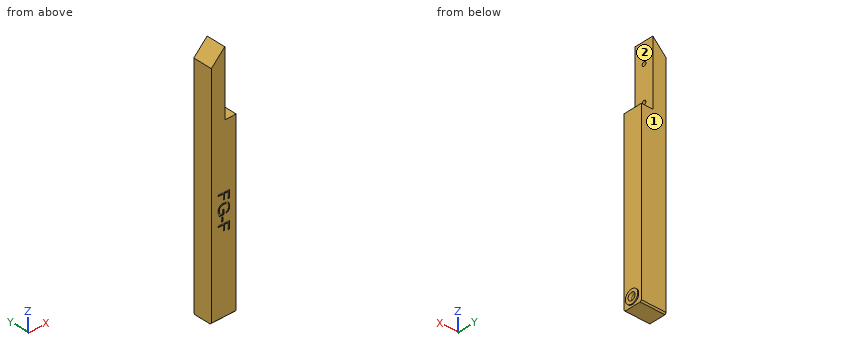
```python
from build123d import *

# Parameters (mm, degrees)
ESQUISSE1_W                         = 13
ESQUISSE1_H                         = 126
BOSS_EXTRU_1_DEPTH                  = 10
ESQUISSE2_W                         = 6
ESQUISSE2_H                         = 34
ENL_V_MAT_EXTRU_1_DEPTH             = 155.389928428
ENL_V_START                         = 1.2
ENL_V_MAT_EXTRU_2_DEPTH             = 0.4
ENL_V_MAT_EXTRU_3_DEPTH             = 0.4
ENL_V_MAT_EXTRU_4_DEPTH             = 0.4
ESQUISSE6_W                         = 0.740791559
ESQUISSE6_H                         = 2.263300419
ENL_V_MAT_EXTRU_5_DEPTH             = 0.4
D_POUILLE1_ANGLE                    = -0.092269995
D_POUILLE2_ANGLE                    = 0.092269995
D_POUILLE3_ANGLE                    = -45
ESQUISSE7_W                         = 0.5
ESQUISSE7_H                         = 3.5
DIAM_TRE_DU_PER_AGE_2_1_2_1_1_D     = 2.1
DIAM_TRE_DU_PER_AGE_2_1_2_1_1_DEPTH = 5
CHANFREIN1_SIZE                     = 0.7


with BuildPart() as part:
    # Esquisse1 → Boss.-Extru.1 (new body)
    with BuildSketch(Plane.XZ.offset(-10)):
        with Locations((21.5, 88.5)):
            Rectangle(ESQUISSE1_W, ESQUISSE1_H)
    extrude(amount=-BOSS_EXTRU_1_DEPTH)

    # Esquisse2 → Enlèv. mat.-Extru.1 (cut, through all)
    with BuildSketch(Plane(origin=(0, 20, 0), x_dir=(-1, 0, 0), z_dir=(0, 1, 0))):
        with Locations((-25, 134.5)):
            Rectangle(ESQUISSE2_W, ESQUISSE2_H)
    extrude(amount=-ENL_V_MAT_EXTRU_1_DEPTH, mode=Mode.SUBTRACT)

    # Esquisse3 → Enlèv. mat.-Extru.2 (cut)
    with BuildSketch(Plane.XZ.offset(-11.2).offset(ENL_V_START)):
        with BuildLine():
            Line((20.853342891, 76.277673701), (21.557298779, 76.278807363))
            Line((21.557298779, 76.278807363), (21.56139183, 73.73719736))
            Line((21.56139183, 73.73719736), (19.337604377, 73.733616136))
            ThreePointArc((19.337604377, 73.733616136), (18.937851016, 74.311477162), (18.633015037, 74.944565734))
            add(Edge.make_bspline(
                [(18.633015037, 74.944565734), (18.598877989, 75.048134715), (18.530815128, 75.254631808), (18.449647927, 75.570941889), (18.41259048, 75.895390829), (18.402660702, 76.11257772), (18.397680402, 76.221508226)],
                knots=[0, 0, 0, 0, 0.250783, 0.500014197, 0.749231153, 1, 1, 1, 1], degree=3))
            add(Edge.make_bspline(
                [(18.397680402, 76.221508226), (18.404707316, 76.360829639), (18.418683348, 76.637930028), (18.475840729, 77.051065085), (18.608033081, 77.446634686), (18.719977562, 77.700354542), (18.776261687, 77.827921352)],
                knots=[0, 0, 0, 0, 0.251459099, 0.500134278, 0.748674478, 1, 1, 1, 1], degree=3))
            add(Edge.make_bspline(
                [(18.776261687, 77.827921352), (18.845594133, 77.939975948), (18.983004533, 78.16205764), (19.226428261, 78.470943979), (19.536080689, 78.713393436), (19.758734474, 78.849811508), (19.871078014, 78.918643436)],
                knots=[0, 0, 0, 0, 0.252300142, 0.500035199, 0.747734736, 1, 1, 1, 1], degree=3))
            add(Edge.make_bspline(
                [(19.871078014, 78.918643436), (19.998387452, 78.973593805), (20.251642055, 79.082905685), (20.645993091, 79.211619983), (21.057113166, 79.266914711), (21.332777469, 79.280276264), (21.471351266, 79.286992988)],
                knots=[0, 0, 0, 0, 0.251271452, 0.499850228, 0.748579513, 1, 1, 1, 1], degree=3))
            add(Edge.make_bspline(
                [(21.471351266, 79.286992988), (21.61250902, 79.279773241), (21.893469007, 79.265403078), (22.312514038, 79.209031831), (22.7157204, 79.081743941), (22.975763595, 78.974547289), (23.106412768, 78.920690259)],
                knots=[0, 0, 0, 0, 0.251233762, 0.500054957, 0.748820933, 1, 1, 1, 1], degree=3))
            add(Edge.make_bspline(
                [(23.106412768, 78.920690259), (23.221187424, 78.855887896), (23.448551437, 78.727517), (23.766911077, 78.49685491), (24.019672726, 78.19573618), (24.162080848, 77.977148745), (24.233970523, 77.866802654)],
                knots=[0, 0, 0, 0, 0.252519074, 0.500230209, 0.747708999, 1, 1, 1, 1], degree=3))
            add(Edge.make_bspline(
                [(24.233970523, 77.866802654), (24.289601824, 77.74114466), (24.400227282, 77.491267832), (24.529493504, 77.101027909), (24.583614751, 76.693519205), (24.596060717, 76.420296572), (24.602319479, 76.282899818)],
                knots=[0, 0, 0, 0, 0.251319556, 0.499760752, 0.748442329, 1, 1, 1, 1], degree=3))
            add(Edge.make_bspline(
                [(24.602319479, 76.282899818), (24.598711263, 76.182464999), (24.591519454, 75.982280772), (24.56051168, 75.683056166), (24.48684006, 75.391387004), (24.423380488, 75.201497819), (24.391541958, 75.106227836)],
                knots=[0, 0, 0, 0, 0.250925915, 0.500139405, 0.749213149, 1, 1, 1, 1], degree=3))
            add(Edge.make_bspline(
                [(24.391541958, 75.106227836), (24.356062424, 75.028126494), (24.285554136, 74.87291611), (24.15898731, 74.650089551), (23.991023414, 74.45654053), (23.86675947, 74.34011923), (23.804229379, 74.281535587)],
                knots=[0, 0, 0, 0, 0.25175747, 0.500316288, 0.748557245, 1, 1, 1, 1], degree=3))
            add(Edge.make_bspline(
                [(23.804229379, 74.281535587), (23.728753924, 74.230590324), (23.578415746, 74.129113387), (23.340086032, 73.996604052), (23.084028963, 73.902840483), (22.909556406, 73.852507456), (22.821965098, 73.827238521)],
                knots=[0, 0, 0, 0, 0.250860638, 0.499684722, 0.748824286, 1, 1, 1, 1], degree=3))
            Line((22.821965098, 73.827238521), (22.625511765, 74.543474159))
            add(Edge.make_bspline(
                [(22.625511765, 74.543474159), (22.689177507, 74.563582686), (22.816125851, 74.603678729), (23.002808274, 74.674933967), (23.178371642, 74.770364118), (23.289904539, 74.84276967), (23.345839262, 74.879081687)],
                knots=[0, 0, 0, 0, 0.250917255, 0.500324495, 0.749408362, 1, 1, 1, 1], degree=3))
            add(Edge.make_bspline(
                [(23.345839262, 74.879081687), (23.390203046, 74.919598808), (23.478372835, 75.000123634), (23.597726044, 75.134487648), (23.688549595, 75.289563684), (23.73964112, 75.397672698), (23.765348077, 75.45206829)],
                knots=[0, 0, 0, 0, 0.251387332, 0.499614011, 0.748228283, 1, 1, 1, 1], degree=3))
            add(Edge.make_bspline(
                [(23.765348077, 75.45206829), (23.789008491, 75.518784077), (23.836150518, 75.651711479), (23.891167257, 75.856395572), (23.914580183, 76.067045865), (23.920133119, 76.208042107), (23.922920108, 76.278807363)],
                knots=[0, 0, 0, 0, 0.250882944, 0.49986997, 0.748987428, 1, 1, 1, 1], degree=3))
            add(Edge.make_bspline(
                [(23.922920108, 76.278807363), (23.920511452, 76.359188387), (23.915711583, 76.519368292), (23.89240824, 76.758868036), (23.834062357, 76.992322036), (23.782857942, 77.144019816), (23.757162571, 77.22014471)],
                knots=[0, 0, 0, 0, 0.251034583, 0.500251096, 0.74921629, 1, 1, 1, 1], degree=3))
            add(Edge.make_bspline(
                [(23.757162571, 77.22014471), (23.729672868, 77.279418984), (23.674945132, 77.397424872), (23.579353438, 77.56786432), (23.456707319, 77.720003547), (23.366562662, 77.813633023), (23.321282744, 77.860663375)],
                knots=[0, 0, 0, 0, 0.25126472, 0.500229098, 0.748963655, 1, 1, 1, 1], degree=3))
            add(Edge.make_bspline(
                [(23.321282744, 77.860663375), (23.275908475, 77.898471307), (23.185404712, 77.973883213), (23.042714988, 78.078444046), (22.887828988, 78.163906132), (22.781260082, 78.214085774), (22.727831483, 78.239243469)],
                knots=[0, 0, 0, 0, 0.250690915, 0.500029454, 0.749338462, 1, 1, 1, 1], degree=3))
            add(Edge.make_bspline(
                [(22.727831483, 78.239243469), (22.630282244, 78.273310635), (22.435887582, 78.341199173), (22.136961191, 78.420956742), (21.82952565, 78.455607579), (21.623732954, 78.464151438), (21.520464301, 78.468438825)],
                knots=[0, 0, 0, 0, 0.250863433, 0.499916891, 0.749053732, 1, 1, 1, 1], degree=3))
            add(Edge.make_bspline(
                [(21.520464301, 78.468438825), (21.404727069, 78.464782543), (21.17444342, 78.457507597), (20.830459066, 78.41956085), (20.498481034, 78.321775426), (20.285218981, 78.235525632), (20.178035378, 78.192177257)],
                knots=[0, 0, 0, 0, 0.251508131, 0.500428504, 0.748919829, 1, 1, 1, 1], degree=3))
            add(Edge.make_bspline(
                [(20.178035378, 78.192177257), (20.095012391, 78.141920052), (19.930593774, 78.042390751), (19.702109128, 77.864604869), (19.524573648, 77.635924233), (19.425752299, 77.47115107), (19.375852227, 77.387948474)],
                knots=[0, 0, 0, 0, 0.252519428, 0.500089146, 0.747568839, 1, 1, 1, 1], degree=3))
            add(Edge.make_bspline(
                [(19.375852227, 77.387948474), (19.337663327, 77.298574803), (19.261671031, 77.120729659), (19.170871606, 76.844534828), (19.129994348, 76.556685787), (19.119293569, 76.36357432), (19.113916039, 76.266528806)],
                knots=[0, 0, 0, 0, 0.251262992, 0.499989565, 0.748726625, 1, 1, 1, 1], degree=3))
            add(Edge.make_bspline(
                [(19.113916039, 76.266528806), (19.118173223, 76.18036823), (19.126657842, 76.008649142), (19.158071405, 75.752276351), (19.226503664, 75.503216877), (19.283711047, 75.341066696), (19.312415004, 75.259707412)],
                knots=[0, 0, 0, 0, 0.250862607, 0.499972264, 0.749109753, 1, 1, 1, 1], degree=3))
            add(Edge.make_bspline(
                [(19.312415004, 75.259707412), (19.340302347, 75.193424583), (19.3959353, 75.061195796), (19.489793739, 74.867464161), (19.606433607, 74.686525861), (19.692748901, 74.572154479), (19.736016273, 74.514823398)],
                knots=[0, 0, 0, 0, 0.250800542, 0.500326436, 0.749528026, 1, 1, 1, 1], degree=3))
            Line((19.736016273, 74.514823398), (20.853342891, 74.514823398))
            Line((20.853342891, 74.514823398), (20.853342891, 76.277673701))
        make_face()
    extrude(amount=-ENL_V_MAT_EXTRU_2_DEPTH, mode=Mode.SUBTRACT)

    # Esquisse4 → Enlèv. mat.-Extru.3 (cut)
    with BuildSketch(Plane.XZ.offset(-10)):
        Polygon((24.500000358, 84.16557475), (18.500000119, 84.16557475), (18.500000119, 83.371577701), (21.225784898, 83.371577701), (21.225784898, 80.555751762), (21.933833838, 80.555751762), (21.933833838, 83.371577701), (23.791950822, 83.371577701), (23.791950822, 80.117825708), (24.500000358, 80.117825708), align=None)
    extrude(amount=-ENL_V_MAT_EXTRU_3_DEPTH, mode=Mode.SUBTRACT)

    # Esquisse5 → Enlèv. mat.-Extru.4 (cut)
    with BuildSketch(Plane.XZ.offset(-10)):
        Polygon((24.500000358, 69.734468898), (18.500000119, 69.734468898), (18.500000119, 68.940470657), (21.225784898, 68.940470657), (21.225784898, 66.124647102), (21.933833838, 66.124647102), (21.933833838, 68.940470657), (23.791950822, 68.940470657), (23.791950822, 65.686719856), (24.500000358, 65.686719856), align=None)
    extrude(amount=-ENL_V_MAT_EXTRU_4_DEPTH, mode=Mode.SUBTRACT)

    # Esquisse6 → Enlèv. mat.-Extru.5 (cut)
    with BuildSketch(Plane.XZ.offset(-10)):
        with Locations((20.671214343, 71.815642556)):
            Rectangle(ESQUISSE6_W, ESQUISSE6_H)
    extrude(amount=-ENL_V_MAT_EXTRU_5_DEPTH, mode=Mode.SUBTRACT)

    # Dépouille1
    d_pouille1_faces = [part.faces().sort_by_distance(p)[0] for p in [
        (20.449498104, 10.2, 73.735406748),
    ]]
    draft(d_pouille1_faces, Plane(origin=(21.680083212, 10.4, 0.034913966), x_dir=(0.0016104145188022617, 0, -0.9999987032816982), z_dir=(-0.9999987032816982, 0, -0.0016104145188022617)), D_POUILLE1_ANGLE)

    # Dépouille2
    d_pouille2_faces = [part.faces().sort_by_distance(p)[0] for p in [
        (21.205320835, 10.2, 76.278240532),
    ]]
    draft(d_pouille2_faces, Plane(origin=(21.680083212, 10.4, 0.034913966), x_dir=(0.0016104145188022617, 0, -0.9999987032816982), z_dir=(-0.9999987032816982, 0, -0.0016104145188022617)), D_POUILLE2_ANGLE)

    # Dépouille3
    d_pouille3_faces = [part.faces().sort_by_distance(p)[0] for p in [
        (18.5, 15, 151.5),
    ]]
    draft(d_pouille3_faces, Plane(origin=(22, 10, 117.5), x_dir=(0, 0, 1), z_dir=(1, 0, 0)), D_POUILLE3_ANGLE)

    # Esquisse7 → Révolution1 (revolve)
    with BuildSketch(Plane.XY.offset(30.000000447), mode=Mode.PRIVATE) as r_volution1_sk:
        with Locations((28.25, 16.750000224)):
            Rectangle(ESQUISSE7_W, ESQUISSE7_H)
    revolve(r_volution1_sk.sketch.rotate(Axis((28, 15.000000224, 30.000000447), (1, 0, 0)), 270), axis=Axis((28, 15.000000224, 30.000000447), (1, 0, 0)))

    # Esquisse8 → Fraisage pour vis à tête fraisée M31 (revolve, cut)
    with BuildSketch(Plane(origin=(28.5, 15.000000224, 30.000000447), x_dir=(0, 0, -1), z_dir=(0, 1, 0))):
        Polygon((0, 0), (0, 7), (1.8, 7), (1.8, 1.5), (2, 0), align=None)
    revolve(axis=Axis((34.85, 15.000000224, 30.000000447), (-1, 0, 0)), mode=Mode.SUBTRACT)

    # Diamètre du perçage Ø2.1 (2.1)1
    with Locations(Plane(origin=(22, 0, 0), x_dir=(0, 0, -1), z_dir=(1, 0, 0))):
        with Locations((-141.000001952, 15.000000224), (-123.000001684, 15.000000224)):
            Hole(DIAM_TRE_DU_PER_AGE_2_1_2_1_1_D / 2, depth=DIAM_TRE_DU_PER_AGE_2_1_2_1_1_DEPTH)

    # Chanfrein1
    chanfrein1_edges = [part.edges().sort_by_distance(p)[0] for p in [
        (21.5, 20, 25.5),
        (21.5, 10, 25.5),
    ]]
    chamfer(chanfrein1_edges, length=CHANFREIN1_SIZE)


solid = part.part
```
Model file for the job. Use its own axes, mm. Face numbers are marked on the shaded views. A direction names the side the tool comes from. Give positions to 0.01 mm unless a question says otherwise; leave off trailing zeros. Order: outer loops, then holes, each group sorted by start corner. A loop starts at its lowest first (then second) coordinate and runs counter-clockwise, first axis right, second up.
1) Pin check, flat tips, straight feed: pin 1 (2 mm diameter, centred on x = 24, y = 15, fed in from +Z); pin 2 (2 mm diameter, centred on y = 13.5, z = 85, fed in from +X); pin 3 (0.6 mm diameter, centred on y = 15, z = 140.5, fed in from +X); pin 4 (0.6 mm diameter, centred on x = 20.5, z = 71.5, fed in from -Y). Stop position of each tip, or through.
2) Wall check: probe 1 along X at (y, z) = (12.25, 76.5); probe 2 along Z at (x, y) = (22.25, 17.5); probe 3 along Y at (x, z) = (21, 69.5). Give the ranges that are in metal, low to high.
3) Saw through at B-B, the plane y = 15. Write the cut outline in (x, z).
4) 3-axis set-ups, long thin cutter, end or side, ignore diameter. For the marked faces 1 and 2: which of +Z, -Z, +X, -X, +Y, -Y reach the whole face in a straight line?
5) Saw through at A-A, the plane x = 25.75. Write the cut outline in (y, z), then the cut area to 3 significant figures.
6) Saw through at C-C, the plane z = 125.5. Write the cut outline in (x, y), then the cut area to 3 significant figures.
Computed:
1. pin 1: stops at z = 117.5
1. pin 2: stops at x = 28
1. pin 3: stops at x = 17
1. pin 4: stops at y = 10
2. probe 1: x = 15 to 28
2. probe 2: z = 25.5 to 117.5
2. probe 3: y = 10.4 to 20
3. outline: (15, 25.5) - (28, 25.5) - (28, 26.5) - (28.5, 26.5) - (28.5, 28) - (27, 28.2) - (21.5, 28.2) - (21.5, 31.8) - (27, 31.8) - (28.5, 32) - (28.5, 33.5) - (28, 33.5) - (28, 117.5) - (22, 117.5) - (22, 121.95) - (17, 121.95) - (17, 124.05) - (22, 124.05) - (22, 139.95) - (17, 139.95) - (17, 142.05) - (22, 142.05) - (22, 151.5) - (15, 144.5) - close
4. face 1: +Z, -Z, +X, -X, +Y
4. face 2: +Z, +X, +Y, -Y
5. outline: (10, 26.2) - (10.7, 25.5) - (19.3, 25.5) - (20, 26.2) - (20, 117.5) - (10, 117.5) - close; hole circle Ø3.6 at (15, 30)
5. area: 909 mm2
6. outline: (15, 10) - (22, 10) - (22, 20) - (15, 20) - close
6. area: 70.0 mm2
